from build123d import *

# Parameters (mm, degrees)
SKETCH_W     = 85
SKETCH_H     = 56
PAD_DEPTH    = 1.6
SKETCH001_R  = 1.4
POCKET_DEPTH = 5
SKETCH002_W  = 17.867575
SKETCH002_H  = 32.844936
PAD001_DEPTH = 14.8
SKETCH003_W  = 21.533829
SKETCH003_H  = 15.952719
PAD002_DEPTH = 13.5
SKETCH004_W  = 18.128704
SKETCH004_H  = 15.222443
PAD003_DEPTH = 1.5
SKETCH005_W  = 8.059815
SKETCH005_H  = 5.559658
PAD004_DEPTH = 4
SKETCH006_W  = 15.403427
SKETCH006_H  = 9.588475
PAD005_DEPTH = 8


with BuildPart() as pad001:
    # Sketch → Pad (new body)
    with BuildSketch(Plane.XY):
        with Locations((-116.737486, 1.084726)):
            Rectangle(SKETCH_W, SKETCH_H)
    extrude(amount=PAD_DEPTH)

    # Sketch001 → Pocket (cut)
    with BuildSketch(Plane.XY.offset(1.6)):
        with Locations((-155.737486, 25.334726)):
            Circle(SKETCH001_R)
        with Locations((-97.737486, 25.334726)):
            Circle(SKETCH001_R)
        with Locations((-97.737486, -23.665274)):
            Circle(SKETCH001_R)
        with Locations((-155.737488, -23.662172)):
            Circle(SKETCH001_R)
    extrude(amount=-POCKET_DEPTH, mode=Mode.SUBTRACT)

    # Sketch002 → Pad001 (new body)
    with BuildSketch(Plane.XY.offset(1.6)):
        with Locations((-81.131173, 10.957084)):
            Rectangle(SKETCH002_W, SKETCH002_H)
    extrude(amount=PAD001_DEPTH)


with BuildPart() as pad004:
    # Pad002 base: copy of Pad001
    add(pad001.part)

    # Sketch003 → Pad002 (new body)
    with BuildSketch(Plane.XY.offset(1.6)):
        with Locations((-82.664124, -16.296502)):
            Rectangle(SKETCH003_W, SKETCH003_H)
    extrude(amount=PAD002_DEPTH)

    # Sketch004 → Pad003 (new body)
    with BuildSketch(Plane(origin=(0, 0, 0), x_dir=(1, 0, 0), z_dir=(0, 0, -1))):
        with Locations((-150.791951, -2.536587)):
            Rectangle(SKETCH004_W, SKETCH004_H)
    extrude(amount=PAD003_DEPTH)

    # Sketch005 → Pad004 (new body)
    with BuildSketch(Plane.XY.offset(1.6)):
        with Locations((-148.477616, -24.671362)):
            Rectangle(SKETCH005_W, SKETCH005_H)
    extrude(amount=PAD004_DEPTH)


with BuildPart() as fusion:
    # Pad005 base: copy of Pad004
    add(pad004.part)

    # Sketch006 → Pad005 (new body)
    with BuildSketch(Plane.XY.offset(1.6)):
        with Locations((-127.049156, -22.703693)):
            Rectangle(SKETCH006_W, SKETCH006_H)
    extrude(amount=PAD005_DEPTH)

    # Fusion: union Pad001, Pad004
    add(pad001.part)
    add(pad004.part)


solid = fusion.part
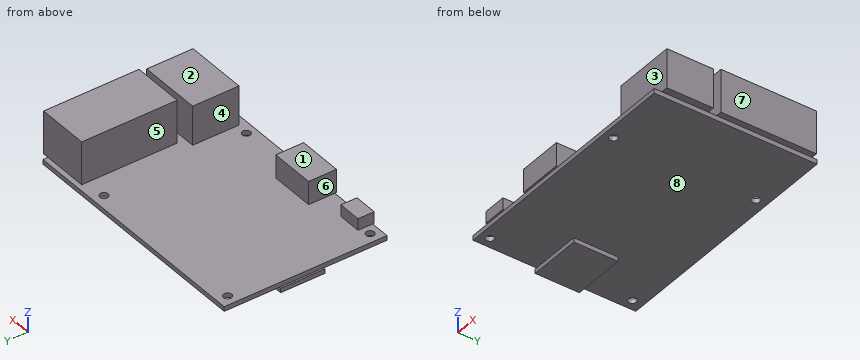
Check sheet for the modelled part. Datum: model origin and axes. Units: mm. Face numbers are marked on the shaded views. A direction names the side the tool comes from. Round coordinates to 2 decimals unless told otherwise and drop trailing zeros. Loops run counter-clockwise (first coordinate to the right, second up) from the corner with the lowest first, then second, coordinate; pieces in that order, holes last. Notation, with made-up numbers: (1, -40) -> (10, -40) arc R25 ccw to (10, -4) -> close; hole circle Ø6 at (10, -19). An arc over 180 degrees is marked (long way). Put each result on its own line as item: value. Start each with the question number.
1. Section check B-B (z = 12). Enter the section's corners in (x, y).
2. Section check C-C (y = -12). Enter the section's corners in (x, z), plus the area to 3 significant figures.
3. Section check D-D (x = -83.5). Enter the section's corners in (y, z).
4. Section check A-A (z = 3.75). Enter the section's corners in (x, y).
5. Draft check along X on the marked faces 6, 7 and 8. Enter one of: +X half, -X half, draft (parallel to the pull), parting line (faces both ways), or undercut.
6. Scan lines: probe 1 along Y at (x, z) = (-83, 12.5); probe 2 along X at (y, z) = (6.5, 6.5); probe 3 along X at (y, z) = (-11, 11.5). Record each from-to range of solid material in increasing order.
7. Access from +Z, -Z, +X, -X, +Y, -Y to the whole of each face (thin tool, end or side, straight path). Record for the marked faces 1, 2, 3, 4 and 5.
8. Gauge pin test, flat ends, axial feed: pin 1 (0.8 mm diameter, centred on y = -11, z = 0.5, fed in from +X); pin 2 (4.5 mm diameter, centred on y = -26, z = 3, fed in from +X); pin 3 (4.5 mm diameter, centred on y = 15, z = 7.5, fed in from +X); pin 4 (4.5 mm diameter, centred on x = -97.74, y = 25.33, fed in from -Z). Record the tip position at first contact, or that the pin passes through.
Findings:
1. outline: (-93.43, -24.27) -> (-71.9, -24.27) -> (-71.9, -8.32) -> (-93.43, -8.32) -> close; (-90.06, -5.47) -> (-72.2, -5.47) -> (-72.2, 27.38) -> (-90.06, 27.38) -> close
2. outline: (-159.24, 0) -> (-74.24, 0) -> (-74.24, 1.6) -> (-71.9, 1.6) -> (-71.9, 15.1) -> (-93.43, 15.1) -> (-93.43, 1.6) -> (-159.24, 1.6) -> close
2. area: 427 mm^2
3. outline: (-26.92, 0) -> (29.08, 0) -> (29.08, 1.6) -> (27.38, 1.6) -> (27.38, 16.4) -> (-5.47, 16.4) -> (-5.47, 1.6) -> (-8.32, 1.6) -> (-8.32, 15.1) -> (-24.27, 15.1) -> (-24.27, 1.6) -> (-26.92, 1.6) -> close
4. outline: (-152.51, -27.45) -> (-144.45, -27.45) -> (-144.45, -21.89) -> (-152.51, -21.89) -> close; (-134.75, -27.5) -> (-119.35, -27.5) -> (-119.35, -17.91) -> (-134.75, -17.91) -> close; (-93.43, -24.27) -> (-71.9, -24.27) -> (-71.9, -8.32) -> (-93.43, -8.32) -> close; (-90.06, -5.47) -> (-72.2, -5.47) -> (-72.2, 27.38) -> (-90.06, 27.38) -> close
5. face 6: undercut
5. face 7: +X half
5. face 8: draft
6. probe 1: y = -24.27 to -8.32, -5.47 to 27.38
6. probe 2: x = -90.06 to -72.2
6. probe 3: x = -93.43 to -71.9
7. face 1: +Z, -X, +Y, -Y
7. face 2: +Z, +X, -X, -Y
7. face 3: +Z, +X, -Y
7. face 4: +Z, +Y, -Y
7. face 5: +Z, -X, +Y
8. pin 1: stops at x = -74.24
8. pin 2: stops at x = -71.9
8. pin 3: stops at x = -72.2
8. pin 4: stops at z = 0
